Drawing for the job (mm, zero at the part's lowest x, y, z). A direction names the side the tool comes from. Give positions to 0.01 mm unless a question says otherwise; leave off trailing zeros. Loops run counter-clockwise (first coordinate to the right, second up) from the corner with the lowest first, then second, coordinate; pieces in that order, holes last. Notation, with made-up numbers: (67.25, 8.5) -> (78.25, 8.5) arc R22 cw to (78.25, 47.5) -> close; hole circle Ø7 at (-6, 7.25). An arc over 180 degrees is marked (long way). Write item = value, one per line.
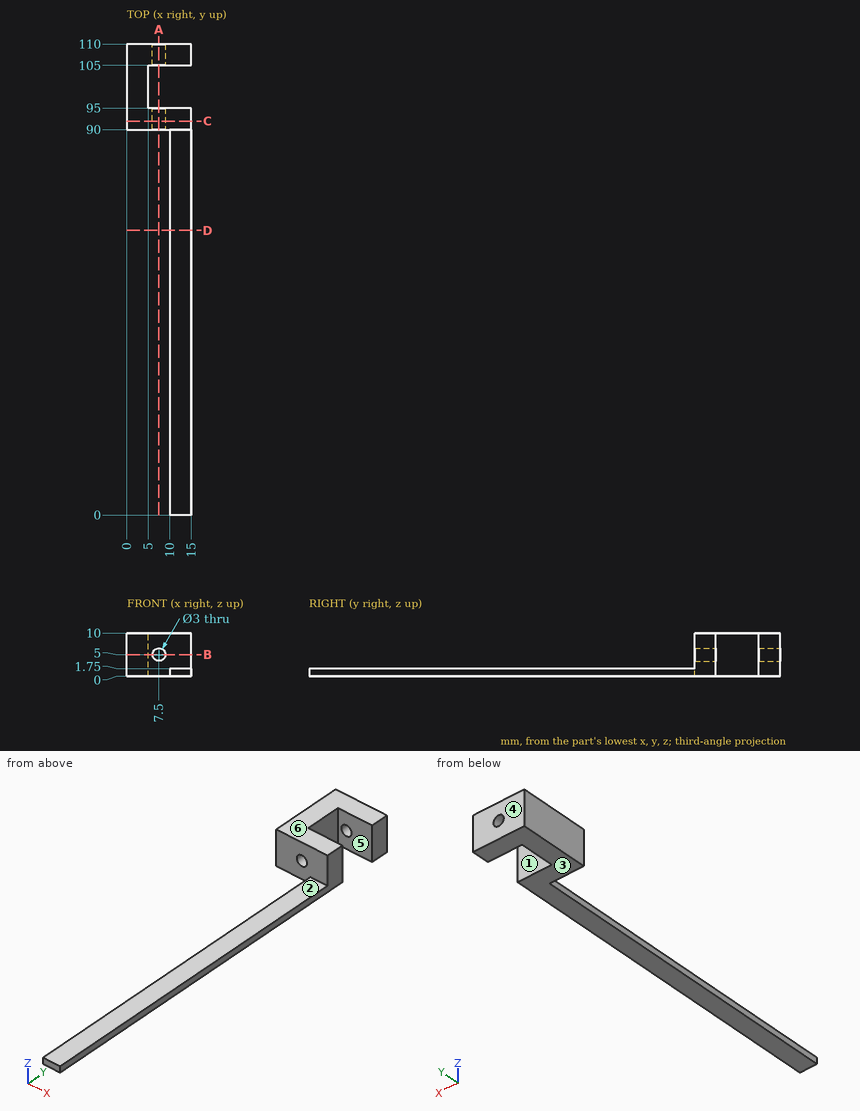
1) Slice it at A-A, the plane x = 7.5. List the corners of the cut face in (y, z).
Resolved:
outline = (90, 0) -> (95, 0) -> (95, 3.5) -> (90, 3.5) -> close; (90, 6.5) -> (95, 6.5) -> (95, 10) -> (90, 10) -> close; (105, 0) -> (110, 0) -> (110, 3.5) -> (105, 3.5) -> close; (105, 6.5) -> (110, 6.5) -> (110, 10) -> (105, 10) -> close
2) Drill centre lines: line 1 along Z through (x, y) = (7.5, 92.5); line 2 along Y through (x, z) = (13.5, 2); line 3 along X through (y, z) = (91.75, 5). Where is each one in solid material? Low to high. Write a range as [from, to].
Resolved:
line_1 = [0, 3.5], [6.5, 10]
line_2 = [90, 95], [105, 110]
line_3 = [0, 6], [9, 15]
3) Drop flat-ended pins along their axis: P1, Ø1, axis at y = 97, z = 2, coming from the +X side; P2, Ø1.9, axis at y = 35, z = 1, coming from the -X side; P3, Ø2, axis at x = 4, z = 8.5, coming from the -Y side; P4, Ø4, axis at y = 49, z = 4.5, coming from the +X side. Give the stop position or say it passes through.
Resolved:
P1 = 5
P2 = 10
P3 = 90
P4 = through
4) Slice it at C-C, the plane y = 92. List the corners of the cut face in (x, z).
Resolved:
outline = (0, 0) -> (15, 0) -> (15, 10) -> (0, 10) -> close; hole circle Ø3 at (7.5, 5)
5) Which spindle directions (+Z, -Z, +X, -X, +Y, -Y) get a long thin tool onto all of the face, cutting with end or side? Do the marked faces 1, 2 and 3. Say none if no direction does.
Resolved:
face_1 = +Z, -Z, +X
face_2 = +Z, +X, -X, -Y
face_3 = -Z, +X, -X, +Y, -Y
6) Slice it at D-D, the plane y = 66.5. List the corners of the cut face in (x, z), and give its area (3 significant figures).
Resolved:
outline = (10, 0) -> (15, 0) -> (15, 1.75) -> (10, 1.75) -> close
area = 8.75 mm²
7) Slice it at B-B, the plane z = 5. List the corners of the cut face in (x, y), and give its area (3 significant figures).
Resolved:
outline = (0, 90) -> (6, 90) -> (6, 95) -> (5, 95) -> (5, 105) -> (6, 105) -> (6, 110) -> (0, 110) -> close; (9, 90) -> (15, 90) -> (15, 95) -> (9, 95) -> close; (9, 105) -> (15, 105) -> (15, 110) -> (9, 110) -> close
area = 170 mm²
8) Pull direction Y, two halves, no side cores. Call the marked faces 4, 5 and 6: pulls with the +Y half, pulls with the -Y half, needs draft (parallel to the pull), parting line crosses it, or undercut.
Resolved:
face_4 = pulls with the +Y half
face_5 = undercut
face_6 = needs draft
